Geometry check sheet. Reference: the model listing, model coordinates, mm. Face numbers are marked on the shaded views. A direction names the side the tool comes from. Coordinates: 2 decimals unless noted, no trailing zeros. Write each loop counter-clockwise with the first axis right and the second up, starting at its lowest first coordinate (ties: lowest second). Pieces come first, ordered by that corner, then holes. Notation, with made-up numbers: (76.5, -36) -> (113.5, -36) arc R20 cw to (113.5, 1) -> close; hole circle Ø1 at (47.25, -33). An arc over 180 degrees is marked (long way). One line per question, with ' | ' between items.
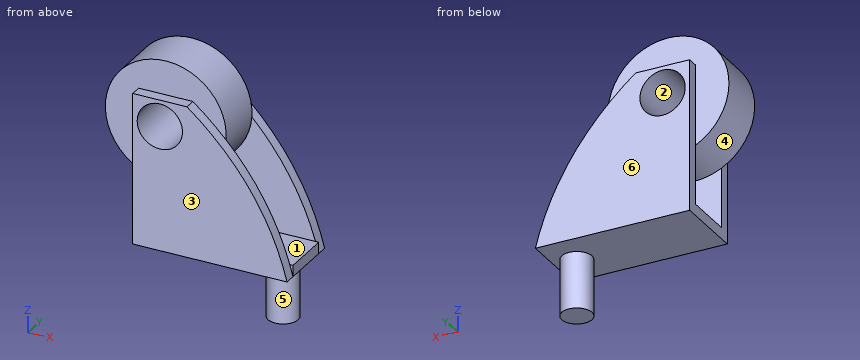
```python
from build123d import *

# Parameters (mm, degrees)
SKETCH_1_R          = 16
SKETCH_1_R_2        = 6
EXTRUDE_1_DEPTH     = 13
EXTRUDE_2_DEPTH     = 3
SKETCH_3_W          = 40.839919316
SKETCH_3_H          = 13
EXTRUDE_3_DEPTH     = 3
SKETCH_4_R          = 4
EXTRUDE_4_DEPTH     = 15
SKETCH_5_R          = 6
CUT_EXTRUDE_1_DEPTH = 30


with BuildPart() as part:
    # 草图1 → 凸台-拉伸1 (new body)
    with BuildSketch(Plane(origin=(0, 0, 0), x_dir=(1, 0, 0), z_dir=(0, 1, 0))):
        with Locations(Location((0, 0, 0), (0, 0, 90))):
            Circle(SKETCH_1_R)
        with Locations(Location((0, 0, 0), (0, 0, 90))):
            Circle(SKETCH_1_R_2, mode=Mode.SUBTRACT)
    extrude(amount=EXTRUDE_1_DEPTH)

    # 草图2 → 凸台-拉伸2 (add)
    with BuildSketch(Plane(origin=(0, 13, 0), x_dir=(1, 0, 0), z_dir=(0, 1, 0))):
        with BuildLine():
            Line((-7.174258512, -6.994775102), (7.174258512, -6.994775102))
            add(Edge.make_bspline(
                [(33.665660804, 33), (27.50458158, 9.184496857), (7.174258512, -6.994775102)],
                knots=[0, 0, 0, 1, 1, 1], degree=2))
            Line((33.665660804, 33), (7.174258512, 33))
            Line((7.174258512, 33), (-7.174258512, 33))
            Line((-7.174258512, 33), (-7.174258512, -6.994775102))
        make_face()
    extrude_2 = extrude(amount=EXTRUDE_2_DEPTH)

    # 镜向1: 凸台-拉伸2 across plane
    add(extrude_2.mirror(Plane.ZX.offset(6.5)))

    # 草图3 → 凸台-拉伸3 (add)
    with BuildSketch(Plane(origin=(0, 0, -33), x_dir=(-1, 0, 0), z_dir=(0, 0, -1))):
        with Locations((-13.245701146, 6.5)):
            Rectangle(SKETCH_3_W, SKETCH_3_H)
    extrude(amount=-EXTRUDE_3_DEPTH)

    # 草图4 → 凸台-拉伸4 (add)
    with BuildSketch(Plane(origin=(0, 0, -33), x_dir=(-1, 0, 0), z_dir=(0, 0, -1))):
        with Locations(Location((-27.665660804, 6.5, 0), (0, 0, 180))):
            Circle(SKETCH_4_R)
    extrude(amount=EXTRUDE_4_DEPTH)

    # 草图5 → 切除-拉伸1 (cut)
    with BuildSketch(Plane.XZ.offset(3)):
        with Locations(Location((0, 0, 0), (0, 0, 270))):
            Circle(SKETCH_5_R)
    extrude(amount=-CUT_EXTRUDE_1_DEPTH, mode=Mode.SUBTRACT)


solid = part.part
```
(1) Material ranges on line 1 (Y direction, x = 3.5, z = -16); line 2 (X direction, y = 6.25, z = 0); line 3 (Z direction, x = 5, y = 2), recorded low to high.
Answers below:
line 1: y = -3 to 0, 13 to 16 | line 2: x = -16 to -6, 6 to 16 | line 3: z = -33 to -30, -15.2 to -3.32, 3.32 to 15.2
(2) Depth check by flat-ended pin: P1, Ø10, axis at y = 11.5, z = -15, coming from the +X side; P2, Ø4, axis at x = 20, y = -0.5, coming from the -Z side; P3, Ø9, axis at x = 1.5, z = 1, coming from the -Y side; P4, Ø1.5, axis at y = 3.5, z = 0, coming from the +X side. Enter the tip coordinate at first touch or a pass-through.
Answers below:
P1: stops at x = 28.87 | P2: stops at z = -33 | P3: stops at y = -3 | P4: stops at x = 16
(3) Cross-section at A-A (x = 0). Record the cut outline in (y, z).
Answers below:
outline: (-3, -33) -> (16, -33) -> (16, -6) -> (-3, -6) -> close; (-3, 6) -> (16, 6) -> (16, 6.99) -> (13, 6.99) -> (13, 16) -> (0, 16) -> (0, 6.99) -> (-3, 6.99) -> close; hole (0, -30) -> (13, -30) -> (13, -16) -> (0, -16) -> close
(4) Draft check along Y on the marked faces 1, 2, 3 and 4. Enter one of: pulls with the +Y half, pulls with the -Y half, needs draft (parallel to the pull), parting line crosses it, or undercut.
Answers below:
face 1: undercut | face 2: needs draft | face 3: pulls with the -Y half | face 4: undercut
(5) Cross-section at B-B (y = 6.5). Record the cut outline in (x, z).
Answers below:
outline: circle Ø32 at (0, 0); (-7.17, -33) -> (23.67, -33) -> (23.67, -48) -> (31.67, -48) -> (31.67, -33) -> (33.67, -33) -> (33.67, -30) -> (-7.17, -30) -> close; hole circle Ø12 at (0, 0)
(6) Cross-section at D-D (z = 9.5). Record the cut outline in (x, y), plus the area to 3 significant figures.
Answers below:
outline: (-12.87, 0) -> (12.87, 0) -> (12.87, 13) -> (-12.87, 13) -> close | area: 335 mm²
(7) Cross-section at C-C (x = -10). Record the cut outline in (y, z).
Answers below:
outline: (0, -12.49) -> (13, -12.49) -> (13, 12.49) -> (0, 12.49) -> close
(8) Tool access check on the marked faces 5 and 6. Record the directions out of +Z, -Z, +X, -X, +Y, -Y that give a thin tool (end or side, any length) a straight path to the whole face; none if there is none.
Answers below:
face 5: -Z | face 6: +Z, -Z, +X, -X, +Y
